Input: part model. Units: mm. Frame: model coordinates. Round coordinates to 2 decimals unless told otherwise and drop trailing zeros. Write each loop counter-clockwise with the first axis right and the second up, starting at its lowest first coordinate (ties: lowest second). Pieces come first, ordered by that corner, then holes. Notation, with made-up numbers: (-13.75, 5) -> (22.25, 5) arc R22 cw to (22.25, 38) -> close; hole circle Ø5 at (72.25, 67). An arc over 180 degrees is marked (long way). Write item = value, one per line.
```python
from build123d import *

# Parameters (mm, degrees)
F0_W     = 15
F0_H     = 15
F1_DEPTH = 2
F3_D     = 1
F4_R     = 1


with BuildPart() as f1:
    # F0 (on Top) → F1 (new body)
    with BuildSketch(Plane.XY):
        with Locations((-7.5, 7.5)):
            Rectangle(F0_W, F0_H)
    extrude(amount=F1_DEPTH)

    # F3 (through all)
    with Locations(Plane.XY.offset(2)):
        with Locations((-7.5, 7.5)):
            Hole(F3_D / 2)

    # F4
    f4_edges = [f1.edges().sort_by_distance(p)[0] for p in [
        (-7.5, 0, 2),
        (-15, 7.5, 2),
        (-7.5, 15, 2),
        (0, 7.5, 2),
        (0, 0, 1),
        (-15, 0, 1),
        (0, 15, 1),
        (-15, 15, 1),
    ]]
    fillet(f4_edges, radius=F4_R)


solid = f1.part
```
1) Line query: L1, parallel to Y at x = -7.5, z = 0.5; L2, parallel to X at y = 3.25, z = 1.65; L3, parallel to X at y = 6, z = 1.2. Output: solid intervals per line, ascending. Write a range as from..to.
Solutions:
L1 = 0..7, 8..15
L2 = -14.76..-0.24
L3 = -14.98..-0.02
2) Cut plane B-B (x = -7.5). Return the cut outline in (y, z), and give its area (3 significant figures).
Solutions:
outline = (0, 0) -> (7, 0) -> (7, 2) -> (1, 2) arc R1 ccw to (0, 1) -> close; (8, 0) -> (15, 0) -> (15, 1) arc R1 ccw to (14, 2) -> (8, 2) -> close
area = 27.6 mm^2
3) Cut plane A-A (y = 7.5). Return the cut outline in (x, z).
Solutions:
outline = (-15, 0) -> (-8, 0) -> (-8, 2) -> (-14, 2) arc R1 ccw to (-15, 1) -> close; (-7, 0) -> (0, 0) -> (0, 1) arc R1 ccw to (-1, 2) -> (-7, 2) -> close
4) Draft query along X for faces 1 (the face through (-14.715, 0.301, 0.507)), 2 (the face through (-7.731, 7.056, 0.986)), 3 (the face through (-0.301, 0.285, 0.507)). Return one class per face: +X half, -X half, draft (parallel to the pull), parting line (faces both ways), or undercut.
Solutions:
face_1 = -X half
face_2 = undercut
face_3 = +X half
5) Cut plane C-C (z = 1.8). Return the cut outline in (x, y), and give its area (3 significant figures).
Solutions:
outline = (-14.6, 1) arc R0.6 ccw to (-14, 0.4) -> (-1, 0.4) arc R0.6 ccw to (-0.4, 1) -> (-0.4, 14) arc R0.6 ccw to (-1, 14.6) -> (-14, 14.6) arc R0.6 ccw to (-14.6, 14) -> close; hole circle Ø1 at (-7.5, 7.5)
area = 201 mm^2
